Autodesk Inventor part; units mm, degrees
ref_plane "Начальная плоскость" through (0, 0, 0) normal (0, 0, 1) x (1, 0, 0)
ref_plane "Конечная плоскость" through (0, 0, 568.945) normal (0, 0, 1) x (1, 0, 0)
ref_plane "РабПлоскость8" through (32.5, 32.5, 568.945) normal (0, 0, 1) x (1, 0, 0)
ref_plane "Начальная плоскость" through (0, 0, 0) normal (0, 0, 1) x (1, 0, 0)
ref_plane "Конечная плоскость" through (0, 0, 568.945) normal (0, 0, 1) x (1, 0, 0)
sketch "Эскиз" plane through (0, 0, 0) normal (0, 0, 1) x (1, 0, 0)
  line L0 (36, -32.5) -> (0, -32.5)
  line L1 (36, -32.5) -> (36, -28.696)
  line L2 (33.6994, -26.2039) -> (9.9215, -24.3017)
  line L3 (4.4, -18.3208) -> (4.4, 18.3208)
  line L4 (33.6994, 26.2039) -> (9.9215, 24.3017)
  line L5 (36, 28.696) -> (36, 32.5)
  line L6 (0, 32.5) -> (36, 32.5)
  line L7 (0, -32.5) -> (0, 32.5)
  arc A0 (4.4, -18.3208) -> (9.9215, -24.3017) centre (10.4, -18.3208) ccw
  arc A1 (9.9215, 24.3017) -> (4.4, 18.3208) centre (10.4, 18.3208) ccw
  arc A2 (36, -28.696) -> (33.6994, -26.2039) centre (33.5, -28.696) ccw
  arc A3 (33.6994, 26.2039) -> (36, 28.696) centre (33.5, 28.696) ccw
  line L8 (0, 45.5) -> (0, -45.5) construction
  line L9 (-7.2974, 0) -> (43.7847, 0) construction
  point P0 (36, -26.388)
  point P1 (4.4, -23.86)
  point P2 (4.4, 23.86)
  point P3 (36, 26.388)
  dimension "d3" = 36
  dimension "d5" = 4.4
  dimension "d7" = 65
  dimension "d9" = 8.64
  dimension "d11" = 8.64
  dimension "d13" = 6.112
  dimension "d15" = 6.112
  dimension "d22" = 6
  dimension "d23" = 2.5
  dimension "d24" = 32.5
  dimension "d25" = 0
extrude "Тело" add sketch "Эскиз" along normal up to surface (568.945 mm away) from surface at 0
sketch "Sketch3" plane through (0, 0, 0) normal (0, 0, 1) x (1, 0, 0)
  line L0 (0, 0) -> (10, 0)
ref_plane "Work Plane7" through (0, 0, 0) normal (0, -1, 0) x (1, 0, 0)
sketch "Sketch4" plane through (0, 0, 0) normal (0, -1, 0) x (1, 0, 0)
  line L0 (-2, 0) -> (12, 0)
  line L1 (-2, 568.945) -> (12, 568.945)
  dimension "d29" = 568.945
ref_plane "РабПлоскость8" through (32.5, 32.5, 568.945) normal (0, 0, 1) x (1, 0, 0)
split "Разделение1" plane through (32.5, 32.5, 568.945) removes the side toward (0, 0, 1)
equation "\"d3\" = b"
equation "\"d7\" = ParH"
equation "\"d22\" = R"
equation "\"d23\" = R1"
equation "\"d24\" = 0.5 * d7"
equation "\"d16\" = G_L"
equation "\"R1\" = 2.5"
equation "\"R\" = 6"
equation "\"t1\" = 4.4"
equation "\"t2\" = 7.2"
equation "\"ParH\" = 65"
equation "\"b\" = 36"
equation "\"msp_x1\" = 0.04 * b"
equation "\"msp_x2\" = -0.08 * t1 + 0.04 * b"
equation "\"G_L\" = d29"
equation "\"ex\" = 0"
equation "\"G_OFFSET_START\" = 0"
equation "\"G_OFFSET_END\" = -36"
equation "\"d27\" = G_OFFSET_END + B_L"
equation "\"B_L\" = 604.945"
properties part number "Швеллер 6.5U-568,95 ГОСТ 8240-97"
Build history of the part. All positions in model axes, mm. A direction names the side the tool comes from. Round coordinates to 2 decimals unless told otherwise and drop trailing zeros. Write each loop counter-clockwise with the first axis right and the second up, starting at its lowest first coordinate (ties: lowest second). Pieces come first, ordered by that corner, then holes. Notation, with made-up numbers: M -3,43.25 L 21,43.25 A25 ccw 21,60.25 Z; hole C 60,54 d6. An arc over 180 degrees is marked long. Answer in a Markdown table with one row per item.
1. Probe L1, parallel to Y at x = 32.5, z = 126.5; L2, parallel to X at y = 18, z = 465; L3, parallel to Y at x = 26, z = 67. List the from-to ranges inside material, lowest first. Write a range as [from, to].
Geometry check:
| item | result |
|---|---|
| L1 | [-32.5, -26.11], [26.11, 32.5] |
| L2 | [0, 4.4] |
| L3 | [-32.5, -25.59], [25.59, 32.5] |
2. Saw through at B-B (x = 26). List the corners of the cut face in (y, z) (3 decimals).
Geometry check:
| item | result |
|---|---|
| outline | M -32.5,0 L -25.588,0 L -25.588,568.945 L -32.5,568.945 Z; M 25.588,0 L 32.5,0 L 32.5,568.945 L 25.588,568.945 Z |
3. Mould opens along Y. For faces 1 (the face through (18, 32.5, 280)), 2 (the face through (4.4, 0, 280)), 3 (the face through (21.977, 25.266, 280.49)), 4 (the face through (0, 0, 280)) say: +Y half, -Y half, draft (parallel to the pull), parting line (faces both ways), or undercut.
Geometry check:
| item | result |
|---|---|
| face 1 | +Y half |
| face 2 | undercut |
| face 3 | undercut |
| face 4 | draft |
4. Which spindle directions (+Z, -Z, +X, -X, +Y, -Y) get a long thin tool onto all of the face, cutting with end or side? Do faces 5 (the face through (21.977, -25.266, 280.49)), 6 (the face through (3, 0, 568.945)). Say none if no direction does.
Geometry check:
| item | result |
|---|---|
| face 5 | +Z, -Z, +X |
| face 6 | +Z, +X, -X, +Y, -Y |
5. Saw through at A-A (z = 493). List the corners of the cut face in (x, y), and give its area (3 significant figures).
Geometry check:
| item | result |
|---|---|
| outline | M 0,-32.5 L 36,-32.5 L 36,-28.7 A2.5 ccw 33.7,-26.2 L 9.92,-24.3 A6 cw 4.4,-18.32 L 4.4,18.32 A6 cw 9.92,24.3 L 33.7,26.2 A2.5 ccw 36,28.7 L 36,32.5 L 0,32.5 Z |
| area | 763 mm2 |
